from build123d import *

# Parameters (mm, degrees)
BOSS_EXTRUDE1_DEPTH = 45.38
SKETCH4_R           = 2.25
CUT_EXTRUDE3_DEPTH  = 14.99956
SKETCH5_R           = 5.54
CUT_EXTRUDE4_DEPTH  = 0.5
CUT_EXTRUDE5_DEPTH  = 2
CUT_EXTRUDE6_DEPTH  = 2
SKETCH2_R           = 2.25
CUT_EXTRUDE7_DEPTH  = 2
SKETCH8_R           = 5.54
CUT_EXTRUDE8_DEPTH  = 1


with BuildPart() as part:
    # Sketch1 → Boss-Extrude1 (new body)
    with BuildSketch(Plane.XY):
        Polygon((-73.15434201, 0), (-73.15434201, -2), (6.88994551, -2), (15.54994551, 12.999559994), (44.34565799, 12.999559994), (44.34565799, 14.999559994), (14.34565799, 14.999559994), (5.68565799, 0), align=None)
    extrude(amount=BOSS_EXTRUDE1_DEPTH)

    # Sketch4 → Cut-Extrude3 (cut)
    with BuildSketch(Plane(origin=(0, 14.999559994, 0), x_dir=(1, 0, 0), z_dir=(0, 1, 0))):
        with Locations((17.34565799, -44.13)):
            Circle(SKETCH4_R)
    cut_extrude3 = extrude(amount=-CUT_EXTRUDE3_DEPTH, mode=Mode.SUBTRACT)

    # Sketch5 → Cut-Extrude4 (cut)
    with BuildSketch(Plane(origin=(0, 14.999559994, 0), x_dir=(1, 0, 0), z_dir=(0, 1, 0))):
        with Locations((17.34565799, -44.13)):
            Circle(SKETCH5_R)
    cut_extrude4 = extrude(amount=-CUT_EXTRUDE4_DEPTH, mode=Mode.SUBTRACT)

    # Sketch6 → Cut-Extrude5 (cut)
    with BuildSketch(Plane(origin=(0, 0, 0), x_dir=(1, 0, 0), z_dir=(0, 1, 0))):
        Polygon((-0.73434201, -36.59), (-0.73434201, -24.824385528), (-6.617149247, -30.707192764), (-33.73434201, -31.053746412), (-33.73434201, -36.59), align=None)
        Polygon((-37.368890626, -36.59), (-37.368890626, -31.053746412), (-31.139529741, -24.824385528), (-58.04173908, -24.824385528), (-64.271099965, -31.053746412), (-64.271099965, -36.59), align=None)
    cut_extrude5 = extrude(amount=-CUT_EXTRUDE5_DEPTH, mode=Mode.SUBTRACT)

    # Sketch7 → Cut-Extrude6 (cut)
    with BuildSketch(Plane(origin=(0, 0, 0), x_dir=(1, 0, 0), z_dir=(0, 1, 0))):
        Polygon((-5.095840943, -22.69), (-6.617149247, -27.890480059), (-25.551142536, -27.890480059), (-29.626528294, -22.69), align=None)
    cut_extrude6 = extrude(amount=-CUT_EXTRUDE6_DEPTH, mode=Mode.SUBTRACT)

    # Sketch2 → Cut-Extrude7 (cut)
    with BuildSketch(Plane(origin=(0, 0, 0), x_dir=(1, 0, 0), z_dir=(0, 1, 0))):
        with Locations((-44.23434201, -44.13)):
            Circle(SKETCH2_R)
    cut_extrude7 = extrude(amount=-CUT_EXTRUDE7_DEPTH, mode=Mode.SUBTRACT)

    # Sketch8 → Cut-Extrude8 (cut)
    with BuildSketch(Plane(origin=(0, 0, 0), x_dir=(1, 0, 0), z_dir=(0, 1, 0))):
        with Locations((-44.23434201, -44.13)):
            Circle(SKETCH8_R)
    cut_extrude8 = extrude(amount=-CUT_EXTRUDE8_DEPTH, mode=Mode.SUBTRACT)

    # Mirror1: Cut-Extrude3, Cut-Extrude4, Cut-Extrude5, Cut-Extrude6, Cut-Extrude7, Cut-Extrude8 across plane
    add(cut_extrude3.mirror(Plane(origin=(0, 0, 22.69), x_dir=(1, 0, 0), z_dir=(0, 0, -1))), mode=Mode.SUBTRACT)
    add(cut_extrude4.mirror(Plane(origin=(0, 0, 22.69), x_dir=(1, 0, 0), z_dir=(0, 0, -1))), mode=Mode.SUBTRACT)
    add(cut_extrude5.mirror(Plane(origin=(0, 0, 22.69), x_dir=(1, 0, 0), z_dir=(0, 0, -1))), mode=Mode.SUBTRACT)
    add(cut_extrude6.mirror(Plane(origin=(0, 0, 22.69), x_dir=(1, 0, 0), z_dir=(0, 0, -1))), mode=Mode.SUBTRACT)
    add(cut_extrude7.mirror(Plane(origin=(0, 0, 22.69), x_dir=(1, 0, 0), z_dir=(0, 0, -1))), mode=Mode.SUBTRACT)
    add(cut_extrude8.mirror(Plane(origin=(0, 0, 22.69), x_dir=(1, 0, 0), z_dir=(0, 0, -1))), mode=Mode.SUBTRACT)


solid = part.part
Could you check a few things on this model? Use its own coordinates, in mm. A direction names the side the tool comes from. Round coordinates to 2 decimals unless told otherwise and drop trailing zeros. Write each loop counter-clockwise with the first axis right and the second up, starting at its lowest first coordinate (ties: lowest second). Pieces come first, ordered by that corner, then holes. Notation, with made-up numbers: (7.5, -24.5) - (56.5, -24.5) arc R18 ccw to (56.5, 2.5) - close; hole circle Ø9 at (-1, -14). An arc over 180 degrees is marked (long way). Put each result on its own line as item: value. Start each with the question number.
(1) I need wall thicknesses on probe 1 along Y at (x, z) = (-9, 37.5); probe 2 along X at (y, z) = (-1.6, 44.13); probe 3 along Y at (x, z) = (27.5, 14). Which ranges of each line are inside material? Lowest first, please.
(2) I want a section at D-D, the plane y = 4. Please give me the cut outline in (x, z), plus the area to 3 significant figures.
(3) I want a section at C-C, the plane x = -2. Please give me the cut outline in (y, z).
(4) Thinking about a two-plate mould opening in Z: for faces 1 (the flat face through (11.159, 5.395, 22.372)), 2 (the flat face through (-9.3, -0.4, 45.38)), 3 (the flat face through (-37.369, -1, 12)), which applies, released by +Z, released by -Z, zero draft, split by the parting line, or undercut?
(5) I want a section at A-A, the plane z = 1.25. Please give me the cut outline in (x, y), plus the area to 3 significant figures.
(6) For faces 4 (the flat face through (32, 14, 0)), 5 (the cylindrical face through (-44.09, -0.49, 38.59)), 6 (the flat face through (-73.154, -1, 22)), 7 (the flat face through (30, 13, 22)), 8 (the flat face through (-3.63, -0.99, 17.66)), which set-ups out of +Z, -Z, +X, -X, +Y, -Y let a thin tool reach every point of the face, with its end or its side?
(7) Will these pins go through, and if not, where does the flat tip stop? pin 1 (8.5 mm diameter, centred on x = 23.5, z = 33.5, fed in from -Y); pin 2 (8 mm diameter, centred on y = 11.5, z = 39.5, fed in from -X); pin 3 (1.6 mm diameter, centred on y = -1.5, z = 34, fed in from +X); pin 4 (1.6 mm diameter, centred on x = -42.5, y = -1, fed in from -Z).
(8) I want a section at B-B, the plane x = -14.5. Please give me the cut outline in (y, z).
Here are the results:
1. probe 1: y = -2 to 0
1. probe 2: x = -73.15 to -46.48, -41.98 to 7.12
1. probe 3: y = 13 to 15
2. outline: (8, 0) - (10.35, 0) - (10.35, 45.38) - (8, 45.38) - close
2. area: 107 mm^2
3. outline: (-2, 0) - (0, 0) - (0, 8.79) - (-2, 8.79) - close; (-2, 19.29) - (0, 19.29) - (0, 26.09) - (-2, 26.09) - close; (-2, 36.59) - (0, 36.59) - (0, 45.38) - (-2, 45.38) - close
4. face 1: zero draft
4. face 2: released by +Z
4. face 3: undercut
5. outline: (-73.15, -2) - (-46.48, -2) - (-46.48, -1) - (-49.77, -1) - (-49.77, 0) - (-73.15, 0) - close; (-41.98, -2) - (6.89, -2) - (15.1, 12.21) - (15.1, 14.5) - (14.06, 14.5) - (5.69, 0) - (-38.69, 0) - (-38.69, -1) - (-41.98, -1) - close; (19.6, 13) - (44.35, 13) - (44.35, 15) - (22.89, 15) - (22.89, 14.5) - (19.6, 14.5) - close
5. area: 226 mm^2
6. face 4: -Z, +X, -X, +Y, -Y
6. face 5: +Y
6. face 6: +Z, -Z, -X, +Y, -Y
6. face 7: +Z, -Z, +X, -Y
6. face 8: +Y, -Y
7. pin 1: stops at y = 13
7. pin 2: stops at x = 10.02
7. pin 3: stops at x = 7.64
7. pin 4: stops at z = 0
8. outline: (-2, 0) - (0, 0) - (0, 8.79) - (-2, 8.79) - close; (-2, 14.57) - (0, 14.57) - (0, 17.49) - (-2, 17.49) - close; (-2, 27.89) - (0, 27.89) - (0, 30.81) - (-2, 30.81) - close; (-2, 36.59) - (0, 36.59) - (0, 45.38) - (-2, 45.38) - close
